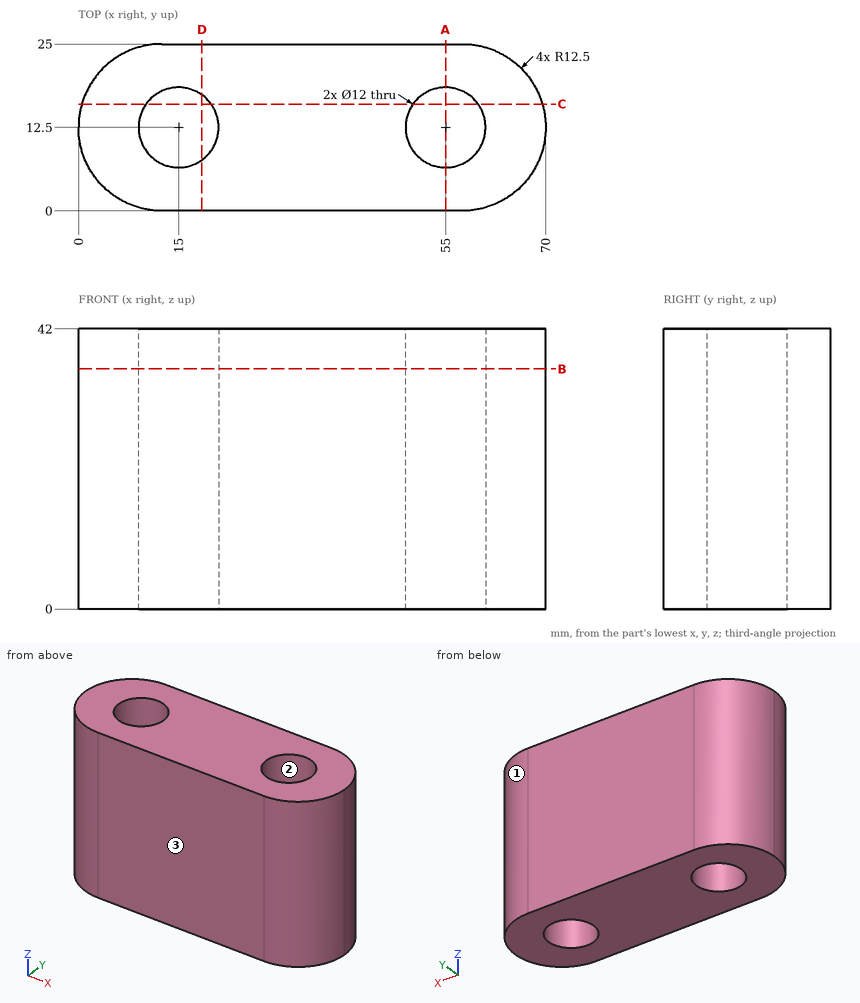
Could you check a few things on this drawing? It's one solid part, dimensions in mm from its lowest x, y, z. Give positions to 0.01 mm unless a question says otherwise; leave off trailing zeros. Order: outer loops, then holes, each group sorted by start corner. A loop starts at its lowest first (then second) coordinate and runs counter-clockwise, first axis right, second up. Notation, with made-up numbers: (76, 82.5) -> (127, 82.5) arc R25 ccw to (127, 103.5) -> close; hole circle Ø7 at (-14.75, -5). An arc over 180 degrees is marked (long way). Answer in a Markdown table with one row per item. Add a question column.
Item 1: We'd pull the mould along X, two halves only. Please class the marked faces 1, 2 and 3: pulls with the +X half, pulls with the -X half, needs draft (parallel to the pull), parting line crosses it, or undercut.
Item 2: Please list where these lines run through material, in increasing order: probe 1 along X at (y, z) = (9, 28); probe 2 along Y at (x, z) = (15, 16); probe 3 along X at (y, z) = (10.75, 18.5).
Item 3: Imagine slicing it at B-B (z = 36). Count the separate pieces of the cut face and the enclosed holes in it, and give its area (3 significant figures).
Item 4: Imagine slicing it at C-C (y = 16). List the corners of the cut face in (x, z) for me.
Item 5: I'm going to push flat-ended pins straight in: P1, Ø3, axis at y = 4.5, z = 8.5, coming from the +X side; P2, Ø7, axis at x = 15, y = 12.5, coming from the +Z side. Where does each tip first touch, or does it pass through?
Item 6: Imagine slicing it at A-A (x = 55). List the corners of the cut face in (y, z) for me.
Item 7: Imagine slicing it at D-D (x = 18.5). List the corners of the cut face in (y, z) for me, and give its area (3 significant figures).
Result:
| question | item | result |
|---|---|---|
| 1 | face 1 | pulls with the +X half |
| 1 | face 2 | undercut |
| 1 | face 3 | needs draft |
| 2 | probe 1 | 0.5 to 10.13, 19.87 to 50.13, 59.87 to 69.5 |
| 2 | probe 2 | 0 to 6.5, 18.5 to 25 |
| 2 | probe 3 | 0.12 to 9.26, 20.74 to 49.26, 60.74 to 69.88 |
| 3 | separate pieces | 1 |
| 3 | enclosed holes | 2 |
| 3 | area | 1,390 mm2 |
| 4 | outline | (0.5, 0) -> (10.13, 0) -> (10.13, 42) -> (0.5, 42) -> close; (19.87, 0) -> (50.13, 0) -> (50.13, 42) -> (19.87, 42) -> close; (59.87, 0) -> (69.5, 0) -> (69.5, 42) -> (59.87, 42) -> close |
| 5 | P1 | x = 68.18 |
| 5 | P2 | through |
| 6 | outline | (0, 0) -> (6.5, 0) -> (6.5, 42) -> (0, 42) -> close; (18.5, 0) -> (25, 0) -> (25, 42) -> (18.5, 42) -> close |
| 7 | outline | (0, 0) -> (7.63, 0) -> (7.63, 42) -> (0, 42) -> close; (17.37, 0) -> (25, 0) -> (25, 42) -> (17.37, 42) -> close |
| 7 | area | 641 mm2 |
